For this review, take the finished solid that the model builds, in its own axes (mm). Face numbers are marked on the shaded views. A direction names the side the tool comes from. Round coordinates to 2 decimals unless told otherwise and drop trailing zeros. Order: outer loops, then holes, each group sorted by start corner. A loop starts at its lowest first (then second) coordinate and runs counter-clockwise, first axis right, second up. Notation, with made-up numbers: M 52.5,53.25 L 58.5,53.25 A27 ccw 58.5,75.25 Z; hole C 26,76.25 d3. An arc over 180 degrees is marked long. Put each result on its own line as item: value.
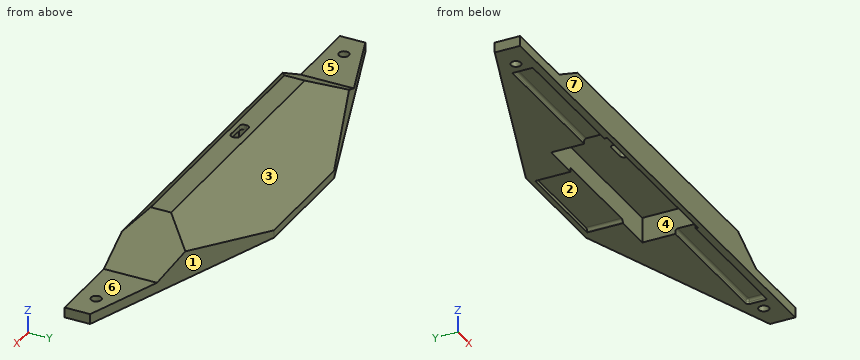
from build123d import *

# Parameters (mm, degrees)
SKETCH002_R       = 2
PAD_DEPTH         = 18
PAD001_DEPTH      = 100
SKETCH007_W       = 40
SKETCH007_H       = 36
PAD004_DEPTH      = 1.5
SKETCH008_W       = 70
SKETCH008_H       = 22
PAD005_DEPTH      = 10
SKETCH009_W       = 56
SKETCH009_H       = 8
PAD006_DEPTH      = 2
SKETCH010_W       = 26.7
SKETCH010_H       = 2.6
PAD007_DEPTH      = 15
PAD008_DEPTH      = 20
PAD008_DEPTH_BACK = 20
SKETCH013_W       = 56
SKETCH013_H       = 8
PAD009_DEPTH      = 2
PAD002_DEPTH      = 120
PAD002_DEPTH_BACK = 120
FILLET_R          = 1
FILLET001_R       = 1
FILLET002_R       = 1
FILLET003_R       = 1
FILLET004_R       = 1


with BuildPart() as body:
    # Sketch002 → Pad (new body)
    with BuildSketch(Plane.XY):
        Polygon((-105.5, -52), (105.5, -52), (105.5, -42), (23.075677, -12), (-23.075677, -12), (-105.5, -42), align=None)
        with Locations((-95, -45)):
            Circle(SKETCH002_R, mode=Mode.SUBTRACT)
        with Locations((95, -45)):
            Circle(SKETCH002_R, mode=Mode.SUBTRACT)
    extrude(amount=PAD_DEPTH)


with BuildPart() as body001:
    # Sketch → Pad001 (new body)
    with BuildSketch(Plane.XZ):
        Polygon((-105.5, 0), (-105.5, 4), (-75.5, 4), (-51.251289, 18), (51.251289, 18), (75.5, 4), (105.5, 4), (105.5, 0), align=None)
    extrude(amount=PAD001_DEPTH)

    # Boolean: intersect Body
    add(body.part, mode=Mode.INTERSECT)


with BuildPart() as body004:
    # Sketch007 → Pad004 (new body)
    with BuildSketch(Plane.XY):
        with Locations((0, -32)):
            Rectangle(SKETCH007_W, SKETCH007_H)
    extrude(amount=PAD004_DEPTH)


with BuildPart() as body005:
    # Sketch008 → Pad005 (new body)
    with BuildSketch(Plane.XY):
        with Locations((0, -39)):
            Rectangle(SKETCH008_W, SKETCH008_H)
    extrude(amount=PAD005_DEPTH)


with BuildPart() as body006:
    # Sketch009 → Pad006 (new body)
    with BuildSketch(Plane.XY):
        with Locations((62, -45)):
            Rectangle(SKETCH009_W, SKETCH009_H)
    extrude(amount=PAD006_DEPTH)


with BuildPart() as body007:
    # Sketch010 → Pad007 (new body)
    with BuildSketch(Plane.XY):
        with Locations((-1.35, -40.3)):
            Rectangle(SKETCH010_W, SKETCH010_H)
    extrude(amount=PAD007_DEPTH)


with BuildPart() as body007_1:
    # Body007 placement: moved
    add(body007.part.moved(Location((0, -3.5, 1))))


with BuildPart() as body008:
    # Sketch011 → Pad008 (new body, two sides)
    with BuildSketch(Plane.XY) as pad008_sk:
        with BuildLine():
            ThreePointArc((-13, -37), (-14.06066, -37.43934), (-14.5, -38.5))
            Line((-14.5, -39.1), (-14.5, -38.5))
            ThreePointArc((-14.5, -39.1), (-14.06066, -40.16066), (-13, -40.6))
            Line((-6.5, -40.6), (-13, -40.6))
            ThreePointArc((-6.5, -40.6), (-5.43934, -40.16066), (-5, -39.1))
            Line((-5, -38.5), (-5, -39.1))
            ThreePointArc((-5, -38.5), (-5.43934, -37.43934), (-6.5, -37))
            Line((-13, -37), (-6.5, -37))
        make_face()
    extrude(amount=PAD008_DEPTH)
    extrude(pad008_sk.sketch, amount=-PAD008_DEPTH_BACK)


with BuildPart() as body008_1:
    # Body008 placement: moved
    add(body008.part.moved(Location((0, -3.5, 11))))


with BuildPart() as body009:
    # Sketch013 → Pad009 (new body)
    with BuildSketch(Plane.XY):
        with Locations((-62, -45)):
            Rectangle(SKETCH013_W, SKETCH013_H)
    extrude(amount=PAD009_DEPTH)


with BuildPart() as back:
    # Sketch003 → Pad002 (new body, two sides)
    with BuildSketch(Plane.YZ) as pad002_sk:
        Polygon((-12, 0), (-12, 3), (-37.980762, 18), (-45.980762, 18), (-52, 11.980762), (-52, 0), align=None)
    extrude(amount=PAD002_DEPTH)
    extrude(pad002_sk.sketch, amount=-PAD002_DEPTH_BACK)

    # Boolean001: intersect Body001
    add(body001.part, mode=Mode.INTERSECT)

    # Boolean002: cut Body004
    add(body004.part, mode=Mode.SUBTRACT)

    # Boolean003: cut Body005
    add(body005.part, mode=Mode.SUBTRACT)

    # Boolean004: cut Body006
    add(body006.part, mode=Mode.SUBTRACT)

    # Boolean005: cut Body007
    add(body007_1.part, mode=Mode.SUBTRACT)

    # Boolean006: cut Body008
    add(body008_1.part, mode=Mode.SUBTRACT)

    # Fillet
    fillet_edges = [back.edges().sort_by_distance(p)[0] for p in [
        (20, -21, 1.5),
    ]]
    fillet(fillet_edges, radius=FILLET_R)

    # Fillet001
    fillet001_edges = [back.edges().sort_by_distance(p)[0] for p in [
        (90, -45, 2),
    ]]
    fillet(fillet001_edges, radius=FILLET001_R)

    # Fillet002
    fillet002_edges = [back.edges().sort_by_distance(p)[0] for p in [
        (62, -41, 2),
    ]]
    fillet(fillet002_edges, radius=FILLET002_R)

    # Fillet003
    fillet003_edges = [back.edges().sort_by_distance(p)[0] for p in [
        (62, -49, 2),
    ]]
    fillet(fillet003_edges, radius=FILLET003_R)

    # Boolean007: cut Body009
    add(body009.part, mode=Mode.SUBTRACT)

    # Fillet004
    fillet004_edges = [back.edges().sort_by_distance(p)[0] for p in [
        (-62.5, -41, 2),
        (-62.5, -49, 2),
        (-90, -45, 2),
    ]]
    fillet(fillet004_edges, radius=FILLET004_R)


solid = back.part
(1) For the marked faces 4, 5, 6 and 7, list the 3-axis set-ups (+Z, -Z, +X, -X, +Y, -Y) from which the entire face can be reached by the end or side of a thin tool; tool diameter is ignored.
A:
face 4: -Z
face 5: +Z, -X, +Y, -Y
face 6: +Z, +X, +Y, -Y
face 7: +Z, -Z, +X, -X, -Y
(2) Add section A-A on x = 3. Give the boundary of the cut face in (y, z).
A:
outline: M -52,0 L -50,0 L -50,10 L -45.1,10 L -45.1,16 L -42.5,16 L -42.5,10 L -28,10 L -28,1.5 L -14,1.5 L -14,0 L -12,0 L -12,3 L -37.98,18 L -45.98,18 L -52,11.98 Z
(3) Add section C-C on y = -24.5. Give the boundary of the cut face in (x, z), then the cut area to 3 significant figures.
A:
outline: M -57.42,0 L -20,0 L -20,1.5 L 19,1.5 A1 cw 20,0.5 L 20,0 L 57.42,0 L 57.42,10.22 L -57.42,10.22 Z
area: 1,110 mm2
(4) Add section B-B on x = 95. Give the boundary of the cut face in (y, z), then the cut area to 3 significant figures.
A:
outline: M -52,0 L -47,0 L -47,4 L -52,4 Z; M -43,0 L -38.18,0 L -38.18,4 L -43,4 Z
area: 39.3 mm2
(5) Draft analysis for pull direction X (two halves, no side actions). For the marked faces 1, 2 and 3, state which applies: released by +X, released by -X, zero draft, split by the parting line, or undercut.
A:
face 1: released by +X
face 2: undercut
face 3: zero draft
(6) Add section D-D on x = -39. Give the boundary of the cut face in (y, z), then the cut area to 3 significant figures.
A:
outline: M -52,0 L -49,0 L -49,1 A1 cw -48,2 L -42,2 A1 cw -41,1 L -41,0 L -17.8,0 L -17.8,6.35 L -37.98,18 L -45.98,18 L -52,11.98 Z
area: 464 mm2
(7) To check wall thickness, follow L1, parallel to X at y = -45, z = 2.75; L2, parallel to X at y = -36, z = 5.25; L3, parallel to Y at x = -95, z = 1.8. State the ranges of each line that lie inside material, in increasing order.
A:
L1: x = -105.5 to -97, -93 to -35, 35 to 93, 97 to 105.5
L2: x = -73.33 to -35, 35 to 73.33
L3: y = -52 to -47, -43 to -38.18
(8) Insertion check: pin 1 Ø3 at (x, y) = (-40, -28) entering from +Z; pin 2 Ø1 at (x, y) = (66, -30) entering from +Z; pin 3 Ø1.8 at (x, z) = (2, 13.5) entering from -Y; pin 4 Ø5 at (x, z) = (-10, 12.5) entering from -Y. Each pin has a flat end and moves straight along its axis. Give the tip position at first contact, or say it passes through.
A:
pin 1: stops at z = 13.1
pin 2: stops at z = 9.77
pin 3: stops at y = -51.38
pin 4: stops at y = -52
